Can you work these out from the model? Positions are in its coordinate system, mm. A direction names the side the tool comes from. Round coordinates to 2 decimals unless told otherwise and drop trailing zeros. Order: outer loops, then holes, each group sorted by start corner. A loop starts at its lowest first (then second) coordinate and runs counter-clockwise, first axis right, second up. Notation, with made-up numbers: M -15,61 L -9,61 A19 cw -9,71 Z; hole C -8.5,38.5 d11. An arc over 180 degrees is marked long. Answer as a JSON object with one key per item and string values. Group by question number.
from build123d import *

# Parameters (mm, degrees)
SKETCH1_R           = 1.3
BOSS_EXTRUDE1_DEPTH = 2.8
SKETCH2_W           = 55.6
SKETCH2_H           = 35.6
SKETCH2_R           = 1.3
BOSS_EXTRUDE2_DEPTH = 3.2
FILLET1_R           = 3
SKETCH4_R           = 19
BOSS_EXTRUDE3_DEPTH = 6
BOSS_EXTRUDE4_DEPTH = 7
SKETCH6_R           = 1.6
CUT_EXTRUDE2_DEPTH  = 14
SKETCH8_R           = 2.8
CUT_EXTRUDE3_DEPTH  = 3.5
BOSS_EXTRUDE5_DEPTH = 6
CUT_EXTRUDE4_REACH  = 8
SKETCH10_W          = 12
SKETCH10_H          = 6.35
SKETCH11_R          = 1.6
CUT_EXTRUDE5_DEPTH  = 10
SKETCH13_R          = 1.6
CUT_EXTRUDE6_DEPTH  = 14
SKETCH14_R          = 2.8
CUT_EXTRUDE7_DEPTH  = 7


with BuildPart() as part:
    # Sketch1 → Boss-Extrude1 (new body)
    with BuildSketch(Plane(origin=(0, 0, 0), x_dir=(1, 0, 0), z_dir=(0, 1, 0))):
        Polygon((-4.5, 17.8), (38.3, 17.8), (38.3, -17.8), (-4.5, -17.8), (-12.2, -17.8), (-17.3, -17.8), (-17.3, 17.8), (-12.2, 17.8), align=None)
        with Locations((-4.5, 15)):
            Circle(SKETCH1_R, mode=Mode.SUBTRACT)
        with Locations((12.5, 15)):
            Circle(SKETCH1_R, mode=Mode.SUBTRACT)
        with Locations((29.5, 15)):
            Circle(SKETCH1_R, mode=Mode.SUBTRACT)
        with Locations((29.5, -15)):
            Circle(SKETCH1_R, mode=Mode.SUBTRACT)
        with Locations((12.5, -15)):
            Circle(SKETCH1_R, mode=Mode.SUBTRACT)
        with Locations((-4.5, -15)):
            Circle(SKETCH1_R, mode=Mode.SUBTRACT)
        Polygon((-4.5, 12.4), (33.2, 12.4), (33.2, -12.4), (-4.5, -12.4), (-12.2, -12.4), (-12.2, 12.4), align=None, mode=Mode.SUBTRACT)
    extrude(amount=BOSS_EXTRUDE1_DEPTH)

    # Sketch2 → Boss-Extrude2 (add)
    with BuildSketch(Plane(origin=(0, 2.8, 0), x_dir=(1, 0, 0), z_dir=(0, 1, 0))):
        with Locations((10.5, 0)):
            Rectangle(SKETCH2_W, SKETCH2_H)
        with Locations((-4.5, -15)):
            Circle(SKETCH2_R, mode=Mode.SUBTRACT)
        with Locations((12.5, -15)):
            Circle(SKETCH2_R, mode=Mode.SUBTRACT)
        with Locations((29.5, -15)):
            Circle(SKETCH2_R, mode=Mode.SUBTRACT)
        with Locations((29.5, 15)):
            Circle(SKETCH2_R, mode=Mode.SUBTRACT)
        with Locations((12.5, 15)):
            Circle(SKETCH2_R, mode=Mode.SUBTRACT)
        with Locations((-4.5, 15)):
            Circle(SKETCH2_R, mode=Mode.SUBTRACT)
        with BuildLine():
            Line((-12.2, 2.722131518), (-12.2, -2.722131518))
            ThreePointArc((-12.2, -2.722131518), (-8.418635414, -9.239944684), (-1.577973384, -12.4))
            Line((-1.577973384, -12.4), (1.577973384, -12.4))
            ThreePointArc((1.577973384, -12.4), (12.5, 0), (1.577973384, 12.4))
            Line((1.577973384, 12.4), (-1.577973384, 12.4))
            ThreePointArc((-1.577973384, 12.4), (-8.418635414, 9.239944684), (-12.2, 2.722131518))
        make_face(mode=Mode.SUBTRACT)
    extrude(amount=BOSS_EXTRUDE2_DEPTH)

    # Fillet1
    fillet1_edges = [part.edges().sort_by_distance(p)[0] for p in [
        (-12.2, 1.4, -12.4),
        (-12.2, 1.4, 12.4),
        (33.2, 1.4, 12.4),
        (33.2, 1.4, -12.4),
    ]]
    fillet(fillet1_edges, radius=FILLET1_R)

    # Sketch4 → Boss-Extrude3 (add)
    with BuildSketch(Plane(origin=(0, 6, 0), x_dir=(1, 0, 0), z_dir=(0, 1, 0))):
        with BuildLine():
            ThreePointArc((-59.656294031, -17.8), (-113.805, 0), (-59.656294031, 17.8))
            Line((-59.656294031, 17.8), (-17.3, 17.8))
            Line((-17.3, 17.8), (-17.3, -17.8))
            Line((-17.3, -17.8), (-59.656294031, -17.8))
        make_face()
        with Locations((-83.805, 0)):
            Circle(SKETCH4_R, mode=Mode.SUBTRACT)
    extrude(amount=-BOSS_EXTRUDE3_DEPTH)

    # Sketch5 → Boss-Extrude4 (add)
    with BuildSketch(Plane.XZ):
        with BuildLine():
            ThreePointArc((-59.656294031, -17.8), (-53.805, 0), (-59.656294031, 17.8))
            ThreePointArc((-59.656294031, 17.8), (-113.805, 0), (-59.656294031, -17.8))
        make_face()
        with BuildLine():
            ThreePointArc((-84.555, 21.036634712), (-104.855, 0), (-84.555, -21.036634712))
            Line((-84.555, -21.036634712), (-84.555, -26.036634712))
            Line((-84.555, -26.036634712), (-83.055, -26.036634712))
            Line((-83.055, -26.036634712), (-83.055, -21.036634712))
            ThreePointArc((-83.055, -21.036634712), (-62.755, 0), (-83.055, 21.036634712))
            Line((-83.055, 21.036634712), (-83.055, 26.036634712))
            Line((-83.055, 26.036634712), (-84.555, 26.036634712))
            Line((-84.555, 26.036634712), (-84.555, 21.036634712))
        make_face(mode=Mode.SUBTRACT)
    extrude(amount=BOSS_EXTRUDE4_DEPTH)

    # Sketch6 → Cut-Extrude2 (cut, through all)
    with BuildSketch(Plane.XZ.offset(7)):
        with Locations((-58.805, 0)):
            Circle(SKETCH6_R)
        with Locations((-71.305, -21.650635095)):
            Circle(SKETCH6_R)
        with Locations((-96.305, -21.650635095)):
            Circle(SKETCH6_R)
        with Locations((-108.805, 0)):
            Circle(SKETCH6_R)
        with Locations((-96.305, 21.650635095)):
            Circle(SKETCH6_R)
        with Locations((-71.305, 21.650635095)):
            Circle(SKETCH6_R)
    extrude(amount=-CUT_EXTRUDE2_DEPTH, mode=Mode.SUBTRACT)

    # Sketch8 → Cut-Extrude3 (cut)
    with BuildSketch(Plane(origin=(0, 6, 0), x_dir=(1, 0, 0), z_dir=(0, 1, 0))):
        with Locations((-96.305, 21.650635095)):
            Circle(SKETCH8_R)
        with Locations((-71.305, 21.650635095)):
            Circle(SKETCH8_R)
        with Locations((-58.805, 0)):
            Circle(SKETCH8_R)
        with Locations((-71.305, -21.650635095)):
            Circle(SKETCH8_R)
        with Locations((-96.305, -21.650635095)):
            Circle(SKETCH8_R)
        with Locations((-108.805, 0)):
            Circle(SKETCH8_R)
    extrude(amount=-CUT_EXTRUDE3_DEPTH, mode=Mode.SUBTRACT)

    # Sketch9 → Boss-Extrude5 (add)
    with BuildSketch(Plane(origin=(0, 6, 0), x_dir=(1, 0, 0), z_dir=(0, 1, 0))):
        with BuildLine():
            Line((-59.656294031, 17.8), (38.3, 17.8))
            Line((38.3, 17.8), (38.3, 30))
            Line((38.3, 30), (-83.805, 30))
            ThreePointArc((-83.805, 30), (-70.277250742, 26.776855678), (-59.656294031, 17.8))
        make_face()
    boss_extrude5 = extrude(amount=-BOSS_EXTRUDE5_DEPTH)

    # Mirror1: Boss-Extrude5 across plane
    add(boss_extrude5.mirror(Plane.XY))

    # Sketch10 → Cut-Extrude4 (cut, up to next)
    with BuildSketch(Plane.XZ, mode=Mode.PRIVATE) as cut_extrude4_sk1:
        with Locations((20.3, -26.825)):
            Rectangle(SKETCH10_W, SKETCH10_H)
    cut_extrude4_tool1 = extrude(cut_extrude4_sk1.sketch, amount=-CUT_EXTRUDE4_REACH, mode=Mode.PRIVATE) & part.part
    add(cut_extrude4_tool1.solids().sort_by_distance((20.3, 0, -26.825))[0], mode=Mode.SUBTRACT)
    # Sketch10 → Cut-Extrude4 (cut, up to next)
    with BuildSketch(Plane.XZ, mode=Mode.PRIVATE) as cut_extrude4_sk2:
        with Locations((-3.7, -26.825)):
            Rectangle(SKETCH10_W, SKETCH10_H)
    cut_extrude4_tool2 = extrude(cut_extrude4_sk2.sketch, amount=-CUT_EXTRUDE4_REACH, mode=Mode.PRIVATE) & part.part
    add(cut_extrude4_tool2.solids().sort_by_distance((-3.7, 0, -26.825))[0], mode=Mode.SUBTRACT)
    # Sketch10 → Cut-Extrude4 (cut, up to next)
    with BuildSketch(Plane.XZ, mode=Mode.PRIVATE) as cut_extrude4_sk3:
        with Locations((-27.7, -26.825)):
            Rectangle(SKETCH10_W, SKETCH10_H)
    cut_extrude4_tool3 = extrude(cut_extrude4_sk3.sketch, amount=-CUT_EXTRUDE4_REACH, mode=Mode.PRIVATE) & part.part
    add(cut_extrude4_tool3.solids().sort_by_distance((-27.7, 0, -26.825))[0], mode=Mode.SUBTRACT)
    # Sketch10 → Cut-Extrude4 (cut, up to next)
    with BuildSketch(Plane.XZ, mode=Mode.PRIVATE) as cut_extrude4_sk4:
        with Locations((-51.7, -26.825)):
            Rectangle(SKETCH10_W, SKETCH10_H)
    cut_extrude4_tool4 = extrude(cut_extrude4_sk4.sketch, amount=-CUT_EXTRUDE4_REACH, mode=Mode.PRIVATE) & part.part
    add(cut_extrude4_tool4.solids().sort_by_distance((-51.7, 0, -26.825))[0], mode=Mode.SUBTRACT)
    # Sketch10 → Cut-Extrude4 (cut, up to next)
    with BuildSketch(Plane.XZ, mode=Mode.PRIVATE) as cut_extrude4_sk5:
        with Locations((20.3, 26.825)):
            Rectangle(SKETCH10_W, SKETCH10_H)
    cut_extrude4_tool5 = extrude(cut_extrude4_sk5.sketch, amount=-CUT_EXTRUDE4_REACH, mode=Mode.PRIVATE) & part.part
    add(cut_extrude4_tool5.solids().sort_by_distance((20.3, 0, 26.825))[0], mode=Mode.SUBTRACT)
    # Sketch10 → Cut-Extrude4 (cut, up to next)
    with BuildSketch(Plane.XZ, mode=Mode.PRIVATE) as cut_extrude4_sk6:
        with Locations((-3.7, 26.825)):
            Rectangle(SKETCH10_W, SKETCH10_H)
    cut_extrude4_tool6 = extrude(cut_extrude4_sk6.sketch, amount=-CUT_EXTRUDE4_REACH, mode=Mode.PRIVATE) & part.part
    add(cut_extrude4_tool6.solids().sort_by_distance((-3.7, 0, 26.825))[0], mode=Mode.SUBTRACT)
    # Sketch10 → Cut-Extrude4 (cut, up to next)
    with BuildSketch(Plane.XZ, mode=Mode.PRIVATE) as cut_extrude4_sk7:
        with Locations((-27.7, 26.825)):
            Rectangle(SKETCH10_W, SKETCH10_H)
    cut_extrude4_tool7 = extrude(cut_extrude4_sk7.sketch, amount=-CUT_EXTRUDE4_REACH, mode=Mode.PRIVATE) & part.part
    add(cut_extrude4_tool7.solids().sort_by_distance((-27.7, 0, 26.825))[0], mode=Mode.SUBTRACT)
    # Sketch10 → Cut-Extrude4 (cut, up to next)
    with BuildSketch(Plane.XZ, mode=Mode.PRIVATE) as cut_extrude4_sk8:
        with Locations((-51.7, 26.825)):
            Rectangle(SKETCH10_W, SKETCH10_H)
    cut_extrude4_tool8 = extrude(cut_extrude4_sk8.sketch, amount=-CUT_EXTRUDE4_REACH, mode=Mode.PRIVATE) & part.part
    add(cut_extrude4_tool8.solids().sort_by_distance((-51.7, 0, 26.825))[0], mode=Mode.SUBTRACT)

    # Sketch11 → Cut-Extrude5 (cut)
    with BuildSketch(Plane.XZ):
        with Locations((-39.7, -26.825)):
            Circle(SKETCH11_R)
        with Locations((-15.7, -26.825)):
            Circle(SKETCH11_R)
        with Locations((8.3, -26.825)):
            Circle(SKETCH11_R)
        with Locations((32.3, -26.825)):
            Circle(SKETCH11_R)
        with Locations((32.3, 26.825)):
            Circle(SKETCH11_R)
        with Locations((8.3, 26.825)):
            Circle(SKETCH11_R)
        with Locations((-15.7, 26.825)):
            Circle(SKETCH11_R)
        with Locations((-39.7, 26.825)):
            Circle(SKETCH11_R)
    extrude(amount=-CUT_EXTRUDE5_DEPTH, mode=Mode.SUBTRACT)

    # Sketch13 → Cut-Extrude6 (cut, through all)
    with BuildSketch(Plane(origin=(0, 6, 0), x_dir=(1, 0, 0), z_dir=(0, 1, 0))):
        with Locations((-104.105177743, -17.033871657)):
            Circle(SKETCH13_R)
        with Locations((-104.105177743, 17.033871657)):
            Circle(SKETCH13_R)
    extrude(amount=-CUT_EXTRUDE6_DEPTH, mode=Mode.SUBTRACT)

    # Sketch14 → Cut-Extrude7 (cut)
    with BuildSketch(Plane.XZ.offset(7)):
        with Locations((-104.105177743, 17.033871657)):
            Circle(SKETCH14_R)
        with Locations((-104.105177743, -17.033871657)):
            Circle(SKETCH14_R)
    extrude(amount=-CUT_EXTRUDE7_DEPTH, mode=Mode.SUBTRACT)


solid = part.part
Item 1: Suppose I cut it at B-B, the plane y = -1.5. State how many separate pieces and enclosed holes the cut face has, and give its area (3 significant figures).
Item 2: If we mould it in two halves opening along Z, with no side actions, what happens to faces 4 (the face through (-22, 6, 0)), 5 (the face through (-28, 3, -23.65)), 6 (the face through (-97.903, -2.317, 21.721))? For each: +Z half, -Z half, draft (parallel to the pull), parting line (faces both ways), or undercut.
Item 3: On a 3-axis mill with a long thin cutter (end or side, diameter ignored), from which of +Z, -Z, +X, -X, +Y, -Y can I reach the whole of each face in a straight line? I mean faces 1 (the face through (14.3, 3, 27)), 2 (the face through (-45.7, 3, -27)), 3 (the face through (-104.71, -3.55, 14.3)). Say none if no direction works.
Item 4: I need wall thicknesses on line 1 (Z direction, x = 29.5, y = 4.25); line 2 (Z direction, x = -15.7, y = 4.85) (3 decimals); line 3 (Z direction, x = 12.5, y = 2.75). Which ranges of each line are inside material? Lowest first, please.
Item 5: Suppose I cut it at A-A, the plane x = -39.7. Write out the boundary of the cut face in (y, z) (3 decimals), and give its area (3 significant figures).
Item 6: Suppose I cut it at D-D, the plane x = 8.3. Write out the boundary of the cut face in (y, z) (3 decimals), and give its area (3 significant figures).
Item 7: I'm going to push flat-ended pins straight in: pin 1 Ø3 at (x, y) = (-27.5, 3.5) entering from +Z; pin 2 Ø3 at (x, z) = (-105, -17) entering from -Y; pin 3 Ø0.8 at (y, z) = (1, -3.5) entering from -X; pin 4 Ø2.5 at (x, z) = (-96.3, 21.65) entering from +Y. Where does each tip first touch, or does it pass through?
Computed:
{
 "1": {"separate pieces": "1", "enclosed holes": "9", "area": "1,320 mm^2"},
 "2": {"face 4": "draft", "face 5": "-Z half", "face 6": "undercut"},
 "3": {"face 1": "+Z, +Y, -Y", "face 2": "-Z, +Y, -Y", "face 3": "-Y"},
 "4": {"line 1": "z = -30 to -16.3, -13.7 to 13.7, 16.3 to 30", "line 2": "z = -30 to -28.425, -25.225 to 25.225, 28.425 to 30", "line 3": "z = -30 to -16.3, -13.7 to -12.4, 12.4 to 13.7, 16.3 to 30"},
 "5": {"outline": "M 0,-30 L 6,-30 L 6,-28.425 L 0,-28.425 Z; M 0,-25.225 L 6,-25.225 L 6,25.225 L 0,25.225 Z; M 0,28.425 L 6,28.425 L 6,30 L 0,30 Z", "area": "322 mm^2"},
 "6": {"outline": "M 0,-30 L 6,-30 L 6,-28.425 L 0,-28.425 Z; M 0,-25.225 L 6,-25.225 L 6,-9.347 L 2.8,-9.347 L 2.8,-12.4 L 0,-12.4 Z; M 0,12.4 L 2.8,12.4 L 2.8,9.347 L 6,9.347 L 6,25.225 L 0,25.225 Z; M 0,28.425 L 6,28.425 L 6,30 L 0,30 Z", "area": "192 mm^2"},
 "7": {"pin 1": "stops at z = 23.65", "pin 2": "stops at y = 0", "pin 3": "stops at x = -113.64", "pin 4": "passes through"}
}
